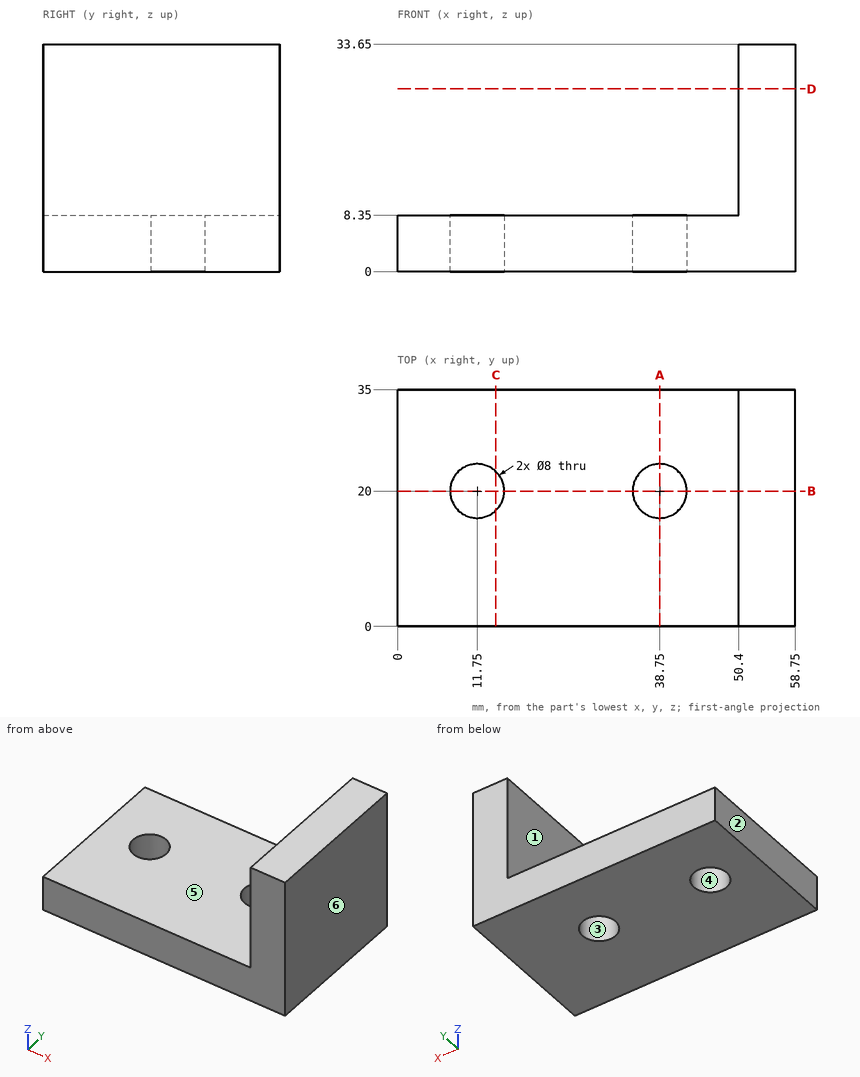
Print and shaded views of the part. All mm, measured from the part's lowest x, y and z. A direction names the side the tool comes from. Coordinates: 2 decimals unless noted, no trailing zeros. Order: outer loops, then holes, each group sorted by start corner. A loop starts at its lowest first (then second) coordinate and runs counter-clockwise, first axis right, second up. Notation, with made-up numbers: (-21.5, 60) - (12.5, 60) arc R27 cw to (12.5, 92) - close; hole circle Ø9 at (-17, -5.5). An arc over 180 degrees is marked (long way). Return JSON: item names as keys, results as strings. Group by question number.
Item 1: Cut at D-D (z = 27). List the corners of the cut face in (x, y), plus the area to 3 significant figures.
Item 2: Cut at B-B (y = 20). List the corners of the cut face in (x, z).
Item 3: Cut at C-C (x = 14.5). List the corners of the cut face in (y, z).
Item 4: Which spindle directions (+Z, -Z, +X, -X, +Y, -Y) get a long thin tool onto all of the face, cutting with end or side? Do the marked faces 1 and 2. Say none if no direction does.
Item 5: Pull direction X, two halves, no side cores. Call the marked faces 3, 4, 5 and 6: pulls with the +X half, pulls with the -X half, needs draft (parallel to the pull), parting line crosses it, or undercut.
Item 6: Pin check, flat tips, straight feed: pin 1 (10.5 mm diameter, centred on x = 22, y = 24.5, fed in from +Z); pin 2 (12 mm diameter, centred on y = 31, z = 17.5, fed in from -X). Stop position of each tip, or through.
Item 7: Cut at A-A (x = 38.75). List the corners of the cut face in (y, z), plus the area to 3 significant figures.
Item 8: Drill centre lines: probe 1 along Y at (x, z) = (38.75, 6.25); probe 2 along X at (y, z) = (22, 7); probe 3 along X at (y, z) = (13, 17.5). Where is each one in solid material? Low to high. Write a range as from..to.
Check values:
{
 "1": {"outline": "(50.4, 0) - (58.75, 0) - (58.75, 35) - (50.4, 35) - close", "area": "292 mm2"},
 "2": {"outline": "(0, 0) - (7.75, 0) - (7.75, 8.35) - (0, 8.35) - close; (15.75, 0) - (34.75, 0) - (34.75, 8.35) - (15.75, 8.35) - close; (42.75, 0) - (58.75, 0) - (58.75, 33.65) - (50.4, 33.65) - (50.4, 8.35) - (42.75, 8.35) - close"},
 "3": {"outline": "(0, 0) - (17.1, 0) - (17.1, 8.35) - (0, 8.35) - close; (22.9, 0) - (35, 0) - (35, 8.35) - (22.9, 8.35) - close"},
 "4": {"face 1": "+Z, -X, +Y, -Y", "face 2": "+Z, -Z, -X, +Y, -Y"},
 "5": {"face 3": "undercut", "face 4": "undercut", "face 5": "needs draft", "face 6": "pulls with the +X half"},
 "6": {"pin 1": "stops at z = 8.35", "pin 2": "stops at x = 50.4"},
 "7": {"outline": "(0, 0) - (16, 0) - (16, 8.35) - (0, 8.35) - close; (24, 0) - (35, 0) - (35, 8.35) - (24, 8.35) - close", "area": "225 mm2"},
 "8": {"probe 1": "y = 0..16, 24..35", "probe 2": "x = 0..8.29, 15.21..35.29, 42.21..58.75", "probe 3": "x = 50.4..58.75"}
}
